The model under review builds one solid part; all positions refer to its coordinate system, in mm. Give positions to 0.01 mm unless a question says otherwise; leave off trailing zeros. Write each loop counter-clockwise with the first axis right and the second up, starting at its lowest first coordinate (ties: lowest second). Pieces come first, ordered by that corner, then holes. Notation, with made-up numbers: (-39, -22.5) - (1, -22.5) arc R3 cw to (1, -17.5) - close; hole circle Ø6 at (47, -5). An arc over 180 degrees is marked (long way). Write item = value, one per line.
```python
from build123d import *

# Parameters (mm, degrees)
F4_R     = 1.5875
F5_DEPTH = 0.79375


# Not quite as in the source:
# - a length typed as a fraction of an inch, garbled in the dataset ("3 / 203.2 mm" for 3/8 in), is restored


with BuildPart() as f2:
    # F2: sweep along a path in F0
    with BuildLine(Plane.XY) as f2_path:
        Line((35.71875, -48.41875), (35.71875, 48.41875))
        Line((35.71875, 48.41875), (-35.71875, 48.41875))
        Line((-35.71875, 48.41875), (-35.71875, -48.41875))
        Line((-35.71875, -48.41875), (35.71875, -48.41875))
    # F1 (on Front) → F2 (sweep)
    with BuildSketch(Plane.XZ):
        with BuildLine():
            Line((31.6033883161, 0.4986022927), (30.95625, 0))
            Line((30.95625, 0), (35.71875, 0))
            Line((35.71875, 0), (35.71875, -3.175))
            Line((35.71875, -3.175), (43.65625, -3.175))
            Line((43.65625, -3.175), (43.65625, 0))
            Line((43.65625, 0), (41.7148061097, 3.175))
            Line((41.7148061097, 3.175), (38.4218543283, 1.8180225684))
            ThreePointArc((38.4218543283, 1.8180225684), (36.4440586883, 1.3544374061), (34.4210724061, 1.5391352618))
            Line((34.4210724061, 1.5391352618), (34.0052636218, 1.6460575328))
            Line((34.0052636218, 1.6460575328), (33.899012953, 1.618762617))
            ThreePointArc((33.899012953, 1.618762617), (32.6942949799, 1.1753032814), (31.6033883161, 0.4986022927))
        make_face()
    sweep(path=f2_path.line, transition=Transition.RIGHT)

    # F4 (on face) → F5 (cut)
    with BuildSketch(Plane(origin=(0, 0, -3.175), x_dir=(1, 0, 0), z_dir=(0, 0, -1))):
        with Locations((-14.5520833333, 52.3875)):
            Circle(F4_R)
        with Locations((0, 52.3875)):
            Circle(F4_R)
        with Locations((14.5520833333, 52.3875)):
            Circle(F4_R)
        with Locations((-14.5520833333, -52.3875)):
            Circle(F4_R)
        with Locations((0, -52.3875)):
            Circle(F4_R)
        with Locations((14.5520833333, -52.3875)):
            Circle(F4_R)
    extrude(amount=-F5_DEPTH, mode=Mode.SUBTRACT)


solid = f2.part
```
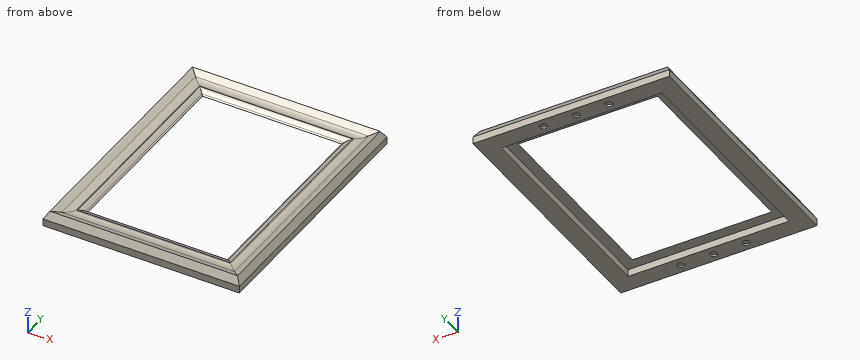
1. For line 1 (Y direction, x = 0, z = -2.95) (3 decimals); line 2 (X direction, y = -31.5, z = -1); line 3 (Y direction, x = -6.5, z = -3), list the stretches that pass through material, from the lowest coordinate up. Write a range as from..to.
Findings below:
line_1 = -56.356..-53.975, -50.8..-48.419, 48.419..50.8, 53.975..56.356
line_2 = -43.66..-35.72, 35.72..43.66
line_3 = -56.36..-48.42, 48.42..56.36
2. Take a section at A-A on y = 34.5. Give the boundary of the cut face in (x, z) (3 decimals), and give its area (3 significant figures).
Findings below:
outline = (-43.656, -3.175) - (-35.719, -3.175) - (-35.719, 0) - (-30.956, 0) - (-31.603, 0.499) arc R6.35 ccw to (-33.899, 1.619) - (-34.005, 1.646) - (-34.421, 1.539) arc R6.35 cw to (-38.422, 1.818) - (-41.715, 3.175) - (-43.656, 0) - close; (30.956, 0) - (35.719, 0) - (35.719, -3.175) - (43.656, -3.175) - (43.656, 0) - (41.715, 3.175) - (38.422, 1.818) arc R6.35 cw to (34.421, 1.539) - (34.005, 1.646) - (33.899, 1.619) arc R6.35 ccw to (31.603, 0.499) - close
area = 92.0 mm²
3. Take a section at C-C on x = -11. Give the boundary of the cut face in (y, z) (3 decimals).
Findings below:
outline = (-56.356, -3.175) - (-48.419, -3.175) - (-48.419, 0) - (-43.656, 0) - (-44.303, 0.499) arc R6.35 ccw to (-46.599, 1.619) - (-46.705, 1.646) - (-47.121, 1.539) arc R6.35 cw to (-51.122, 1.818) - (-54.415, 3.175) - (-56.356, 0) - close; (43.656, 0) - (48.419, 0) - (48.419, -3.175) - (56.356, -3.175) - (56.356, 0) - (54.415, 3.175) - (51.122, 1.818) arc R6.35 cw to (47.121, 1.539) - (46.705, 1.646) - (46.599, 1.619) arc R6.35 ccw to (44.303, 0.499) - close
4. Insertion check: P1, Ø3, axis at x = 34.5, z = 2, coming from the -Y side; P2, Ø4, axis at x = 14.55, y = 52.39, coming from the +Z side; P3, Ø2.5, axis at x = 0.5, y = -52, coming from the -Z side (3 decimals); P4, Ø3, axis at x = 0, y = -52.39, coming from the -Z side. Each pin has a flat end and moves straight along its axis. Give the tip position at first contact, or say it passes through.
Findings below:
P1 = -56.05
P2 = 3.16
P3 = -3.175
P4 = -2.38
